```python
from build123d import *

# Parameters (mm, degrees)
SKETCH1_W           = 20
SKETCH1_H           = 10
BOSS_EXTRUDE1_DEPTH = 130
SKETCH2_R           = 3
CUT_EXTRUDE1_DEPTH  = 140
CUT_EXTRUDE2_DEPTH  = 4
LPATTERN1_COUNT     = 2
LPATTERN1_PITCH     = 60
SKETCH4_W           = 6
SKETCH4_H           = 1.5
CUT_EXTRUDE3_DEPTH  = 200
CHAMFER1_SIZE       = 0.5


with BuildPart() as part:
    # Sketch1 → Boss-Extrude1 (new body)
    with BuildSketch(Plane.XY):
        with Locations((10, 15.187969925)):
            Rectangle(SKETCH1_W, SKETCH1_H)
    extrude(amount=BOSS_EXTRUDE1_DEPTH)

    # Sketch2 → Cut-Extrude1 (cut)
    with BuildSketch(Plane(origin=(0, 20.187969925, 0), x_dir=(1, 0, 0), z_dir=(0, 1, 0))):
        with Locations((12.5, -35)):
            Circle(SKETCH2_R)
    cut_extrude1 = extrude(amount=-CUT_EXTRUDE1_DEPTH, mode=Mode.SUBTRACT)

    # Sketch3 → Cut-Extrude2 (cut)
    with BuildSketch(Plane(origin=(0, 20.187969925, 0), x_dir=(1, 0, 0), z_dir=(0, 1, 0))):
        Polygon((12.5, -29.803847577), (8, -32.401923789), (8, -37.598076211), (12.5, -40.196152423), (17, -37.598076211), (17, -32.401923789), align=None)
    cut_extrude2 = extrude(amount=-CUT_EXTRUDE2_DEPTH, mode=Mode.SUBTRACT)

    # LPattern1: Cut-Extrude1, Cut-Extrude2 ×2
    with Locations(*[(0, 0, i * LPATTERN1_PITCH) for i in range(1, LPATTERN1_COUNT)]):
        add(cut_extrude1, mode=Mode.SUBTRACT)
        add(cut_extrude2, mode=Mode.SUBTRACT)

    # Sketch4 → Cut-Extrude3 (cut)
    with BuildSketch(Plane(origin=(0, 0, 0), x_dir=(-1, 0, 0), z_dir=(0, 0, -1))):
        with Locations((-3, 10.937969925)):
            Rectangle(SKETCH4_W, SKETCH4_H)
    extrude(amount=-CUT_EXTRUDE3_DEPTH, mode=Mode.SUBTRACT)

    # Chamfer1
    chamfer1_edges = [part.edges().sort_by_distance(p)[0] for p in [
        (9.5, 10.187969925, 35),
        (14.75, 20.187969925, 31.102885683),
        (10.25, 20.187969925, 31.102885683),
        (8, 20.187969925, 35),
        (10.25, 20.187969925, 38.897114317),
        (14.75, 20.187969925, 38.897114317),
        (17, 20.187969925, 35),
        (9.5, 10.187969925, 95),
        (14.75, 20.187969925, 91.102885683),
        (10.25, 20.187969925, 91.102885683),
        (8, 20.187969925, 95),
        (10.25, 20.187969925, 98.897114317),
        (14.75, 20.187969925, 98.897114317),
        (17, 20.187969925, 95),
        (10, 20.187969925, 0),
        (13, 10.187969925, 0),
        (13, 10.187969925, 130),
        (6, 10.187969925, 65),
        (20, 10.187969925, 65),
        (0, 20.187969925, 65),
        (20, 20.187969925, 65),
        (10, 20.187969925, 130),
    ]]
    chamfer(chamfer1_edges, length=CHAMFER1_SIZE)


solid = part.part
```
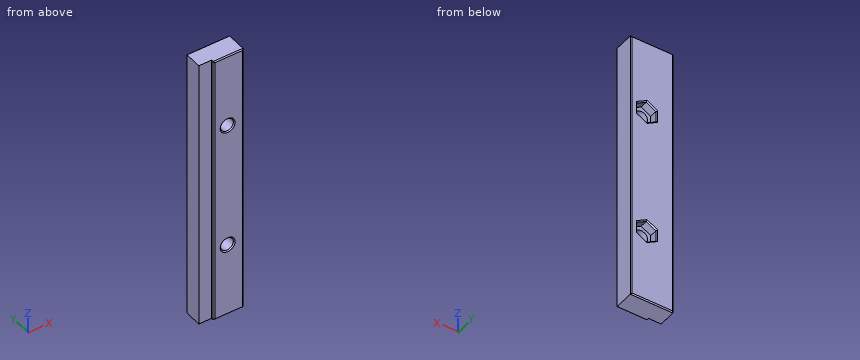
Check sheet for the modelled part. Datum: model origin and axes. Units: mm. Round coordinates to 2 decimals unless told otherwise and drop trailing zeros. Order: outer loops, then holes, each group sorted by start corner. A loop starts at its lowest first (then second) coordinate and runs counter-clockwise, first axis right, second up. Notation, with made-up numbers: (6.25, 83) - (27.25, 83) arc R32 ccw to (27.25, 116) - close; hole circle Ø1 at (-27, -19). An arc over 180 degrees is marked (long way). Answer as CSV lines item,"result". Start each with the question number.
1) Section check A-A (z = 95). Record the cut outline in (x, y).
2) Section check C-C (z = 110). Record the cut outline in (x, y).
3) Section check B-B (y = 17.25). Record the cut outline in (x, z).
4) Scan lines: probe 1 along Z at (x, y) = (12.5, 14.75); probe 2 along X at (y, z) = (15.1, 95); probe 3 along Z at (x, y) = (8.25, 18). Record each from-to range of solid material in increasing order.
5) Depth check by flat-ended pin: pin 1 (4.5 mm diameter, centred on x = 13.5, z = 93.5, fed in from +Y); pin 2 (1 mm diameter, centred on x = 4, z = 83, fed in from -Y). Enter the tip coordinate at first touch or a pass-through.
Determined:
1,outline,"(0, 11.69) - (6, 11.69) - (6, 10.69) - (6.5, 10.19) - (9, 10.19) - (9.5, 10.69) - (9.5, 16.19) - (8, 16.19) - (8, 19.69) - (7.5, 20.19) - (0.5, 20.19) - (0, 19.69) - close; (15.5, 10.69) - (16, 10.19) - (19.5, 10.19) - (20, 10.69) - (20, 19.69) - (19.5, 20.19) - (17.5, 20.19) - (17, 19.69) - (17, 16.19) - (15.5, 16.19) - close"
2,outline,"(0, 11.69) - (6, 11.69) - (6, 10.69) - (6.5, 10.19) - (19.5, 10.19) - (20, 10.69) - (20, 19.69) - (19.5, 20.19) - (0.5, 20.19) - (0, 19.69) - close"
3,outline,"(0, 0) - (20, 0) - (20, 130) - (0, 130) - close; hole (8, 32.4) - (12.5, 29.8) - (17, 32.4) - (17, 37.6) - (12.5, 40.2) - (8, 37.6) - close; hole (8, 92.4) - (12.5, 89.8) - (17, 92.4) - (17, 97.6) - (12.5, 100.2) - (8, 97.6) - close"
4,probe 1,"0 to 32, 38 to 92, 98 to 130"
4,probe 2,"0 to 9.5, 15.5 to 20"
4,probe 3,"0 to 32.26, 37.74 to 92.26, 97.74 to 130"
5,pin 1,"y = 16.19"
5,pin 2,"y = 11.69"
